from build123d import *

# Parameters (mm, degrees)
BOSS_EXTRUDE1_DEPTH = 30
BOSS_EXTRUDE2_START = -3
SKETCH2_R           = 2.5
BOSS_EXTRUDE2_DEPTH = 3
SKETCH3_R           = 2
CUT_EXTRUDE1_DEPTH  = 42.638807138
SKETCH3_4_R         = 3
SKETCH3_4_R_2       = 2
CUT_EXTRUDE7_DEPTH  = 17
FILLET1_R           = 10


with BuildPart() as part:
    # Sketch1 → Boss-Extrude1 (new body)
    with BuildSketch(Plane.XY):
        with BuildLine():
            Line((-20.827632123, 20), (0, 20))
            Line((0, 20), (0, 12.5))
            ThreePointArc((0, 12.5), (-12.5, 0), (0, -12.5))
            Line((0, -12.5), (0, -20))
            Line((0, -20), (-20.827632123, -20))
            Line((-20.827632123, -20), (-20.827632123, 20))
        make_face()
    extrude(amount=BOSS_EXTRUDE1_DEPTH)

    # Sketch2 → Boss-Extrude2 (add)
    with BuildSketch(Plane.XY.offset(30).offset(BOSS_EXTRUDE2_START)):
        with BuildLine():
            Line((0, 12.5), (0, 3))
            ThreePointArc((0, 3), (-3, 0), (0, -3))
            Line((0, -3), (0, -12.5))
            ThreePointArc((0, -12.5), (-12.5, 0), (0, 12.5))
        make_face()
        with Locations((-8.5, 0)):
            Circle(SKETCH2_R, mode=Mode.SUBTRACT)
    extrude(amount=BOSS_EXTRUDE2_DEPTH)

    # Sketch3 → Cut-Extrude1 (cut, through all)
    with BuildSketch(Plane(origin=(0, 0, 0), x_dir=(0, 0, -1), z_dir=(1, 0, 0))):
        with Locations(Location((-20, 0, 0), (0, 0, 90))):
            Circle(SKETCH3_R)
        with Locations(Location((-5, 0, 0), (0, 0, 90))):
            Circle(SKETCH3_R)
    extrude(amount=-CUT_EXTRUDE1_DEPTH, mode=Mode.SUBTRACT)

    # Sketch3_4 → Cut-Extrude7 (cut)
    # profile 1 of 2: a face of its own
    with BuildSketch(Plane(origin=(0, 0, 0), x_dir=(0, 0, -1), z_dir=(1, 0, 0))):
        with Locations(Location((-5, 0, 0), (0, 0, 90))):
            Circle(SKETCH3_4_R)
        with Locations(Location((-5, 0, 0), (0, 0, 90))):
            Circle(SKETCH3_4_R_2, mode=Mode.SUBTRACT)
    # profile 2 of 2: a face of its own
    with BuildSketch(Plane(origin=(0, 0, 0), x_dir=(0, 0, -1), z_dir=(1, 0, 0))):
        with Locations(Location((-20, 0, 0), (0, 0, 90))):
            Circle(SKETCH3_4_R)
        with Locations(Location((-20, 0, 0), (0, 0, 90))):
            Circle(SKETCH3_4_R_2, mode=Mode.SUBTRACT)
    extrude(amount=-CUT_EXTRUDE7_DEPTH, mode=Mode.SUBTRACT)

    # Fillet1
    fillet1_edges = [part.edges().sort_by_distance(p)[0] for p in [
        (-20.827632123, -20, 15),
        (-20.827632123, 20, 15),
    ]]
    fillet(fillet1_edges, radius=FILLET1_R)


solid = part.part
Read the model definition and answer for the solid it produces. Units are mm, in the model's axes. A direction names the side the tool comes from. Give positions to 0.01 mm unless a question says otherwise; leave off trailing zeros. Write each loop counter-clockwise with the first axis right and the second up, starting at its lowest first coordinate (ties: lowest second). Pieces come first, ordered by that corner, then holes. Notation, with made-up numbers: (-26.75, 18) - (29.25, 18) arc R17 cw to (29.25, 34) - close; hole circle Ø3 at (-19.75, 86.5). An arc over 180 degrees is marked (long way). Use CSV: the item, a comma, the result in double quotes. Start each with the question number.
(1) Find section B-B (y = 0). Give the vertices of the cut face in (x, z), plus the area to 3 significant figures.
(2) For faces 1 (the flat face through (0, -15, 15)), 2 (the cylindrical face through (-12.497, 0.275, 13.311)), 3 (the cylindrical face through (-15, -3, 20)), determine the directions among +Z, -Z, +X, -X, +Y, -Y from which every point of the face is accessible in a straight line to the end or side of a thin tool.
(3) Find section D-D (x = -10.25). Give the vertices of the cut face in (y, z).
(4) Determine the mould class of faces 4 (the cylindrical face through (-15, -3, 5)), 5 (the cylindrical face through (-11, 0, 28)), 6 (the flat face through (-13, 0, 0)) for opening direction Z: +Z half, -Z half, draft (parallel to the pull), parting line (faces both ways), or undercut.
(5) Given P1, Ø8, axis at x = -16.5, z = 12.5, coming from the +Y side; P2, Ø6.5, axis at y = -0.5, z = 20.5, coming from the +X side; P3, Ø3.5, axis at y = 0, z = 5, coming from the +X side; P4, Ø3, axis at y = 1, z = 4, coming from the +X side, each flat-ended and moving along its own axis, determine where each tip first touches the part or whether it passes through.
(6) Find section A-A (z = 5). Give the vertices of the cut face in (x, y).
(7) Consider line 1 along Z through (x, y) = (-13.35, 0); line 2 along Y through (x, z) = (-8.5, 28); line 3 along Z through (x, y) = (-20.1, 0). Determine where each line is inside the solid, lowest interval first.
(8) Find section C-C (z = 25). Give the vertices of the cut face in (x, y), plus the area to 3 significant figures.
Findings below:
1,outline,"(-20.83, 0) - (-12.5, 0) - (-12.5, 2) - (-17, 2) - (-17, 3) - (-20.83, 3) - close; (-20.83, 7) - (-17, 7) - (-17, 8) - (-12.5, 8) - (-12.5, 17) - (-17, 17) - (-17, 18) - (-20.83, 18) - close; (-20.83, 22) - (-17, 22) - (-17, 23) - (-12.5, 23) - (-12.5, 27) - (-11, 27) - (-11, 30) - (-20.83, 30) - close; (-6, 27) - (-3, 27) - (-3, 30) - (-6, 30) - close"
1,area,"179 mm2"
2,face 1,"+Z, -Z, +X, +Y, -Y"
2,face 2,"-Z, +X"
2,face 3,"+X"
3,outline,"(-20, 0) - (-7.15, 0) - (-7.15, 27) - (-1.79, 27) - (-1.79, 30) - (-20, 30) - close; (1.79, 27) - (7.15, 27) - (7.15, 0) - (20, 0) - (20, 30) - (1.79, 30) - close"
4,face 4,"undercut"
4,face 5,"draft"
4,face 6,"-Z half"
5,P1,"y = 19.86"
5,P2,"x = -11.92"
5,P3,"through"
5,P4,"x = -17"
6,outline,"(-20.83, -10) arc R10 ccw to (-10.83, -20) - (0, -20) - (0, -12.5) arc R12.5 cw to (-12.13, -3) - (-17, -3) - (-17, -2) - (-20.83, -2) - close; (-20.83, 2) - (-17, 2) - (-17, 3) - (-12.13, 3) arc R12.5 cw to (0, 12.5) - (0, 20) - (-10.83, 20) arc R10 ccw to (-20.83, 10) - close"
7,line 1,"0 to 2, 8 to 17, 23 to 30"
7,line 2,"-20 to -2.5, 2.5 to 20"
7,line 3,"0 to 3, 7 to 18, 22 to 30"
8,outline,"(-20.83, -10) arc R10 ccw to (-10.83, -20) - (0, -20) - (0, -12.5) arc R12.5 cw to (0, 12.5) - (0, 20) - (-10.83, 20) arc R10 ccw to (-20.83, 10) - close"
8,area,"545 mm2"
